For this review, take the finished solid that the model builds, in its own axes (mm). Face numbers are marked on the shaded views. A direction names the side the tool comes from. Coordinates: 2 decimals unless noted, no trailing zeros. Loops run counter-clockwise (first coordinate to the right, second up) from the corner with the lowest first, then second, coordinate; pieces in that order, holes last. Notation, with made-up numbers: (57.25, -14) -> (74.25, -14) arc R26 cw to (74.25, 4) -> close; hole circle Ø1 at (45, 57.5). An arc over 180 degrees is marked (long way). One line per item, written item: value.
from build123d import *

# Parameters (mm, degrees)
SKETCH1_W                   = 82.55
SKETCH1_H                   = 69.85
BOSS_EXTRUDE1_DEPTH         = 19.05
F_3_8_CLEARANCE_HOLE1_D     = 10.31875
F_3_8_CLEARANCE_HOLE1_DEPTH = 38.1
F_3_8_CLEARANCE_HOLE1_TIP   = 3.100065256
F_3_8_CLEARANCE_HOLE2_D     = 10.31875
F_3_8_CLEARANCE_HOLE2_DEPTH = 38.1
F_3_8_CLEARANCE_HOLE2_TIP   = 3.100065256
CUT_EXTRUDE2_START          = -19.05
SKETCH6_R                   = 7.3421875
CUT_EXTRUDE2_DEPTH          = 28.448
CUT_EXTRUDE4_START          = -19.05
SKETCH7_R                   = 12.7254
CUT_EXTRUDE4_DEPTH          = 2.8194
CUT_EXTRUDE6_START          = -19.05
SKETCH8_R                   = 7.3421875
CUT_EXTRUDE6_DEPTH          = 28.448
CUT_EXTRUDE8_START          = -19.05
SKETCH9_R                   = 12.7254
CUT_EXTRUDE8_DEPTH          = 2.8194
CUT_EXTRUDE10_START         = 41.275
SKETCH10_R                  = 7.3421875
CUT_EXTRUDE10_DEPTH         = 60.452


with BuildPart() as part:
    # Sketch1 → Boss-Extrude1 (new, symmetric)
    with BuildSketch(Plane(origin=(0, 0, 0), x_dir=(0, 1, 0), z_dir=(0, 0, 1))):
        Rectangle(SKETCH1_W, SKETCH1_H)
    extrude(amount=BOSS_EXTRUDE1_DEPTH, both=True)

    # 3/8 Clearance Hole1
    with Locations(Plane(origin=(0, 0, -19.05), x_dir=(-1, 0, 0), z_dir=(0, 0, -1))):
        with Locations((-23.876, -30.226)):
            Hole(F_3_8_CLEARANCE_HOLE1_D / 2, depth=F_3_8_CLEARANCE_HOLE1_DEPTH)
            with Locations((0, 0, -(F_3_8_CLEARANCE_HOLE1_DEPTH + F_3_8_CLEARANCE_HOLE1_TIP / 2))):  # 118° drill point
                Cone(0, F_3_8_CLEARANCE_HOLE1_D / 2, F_3_8_CLEARANCE_HOLE1_TIP, mode=Mode.SUBTRACT)

    # 3/8 Clearance Hole2
    with Locations(Plane(origin=(0, 0, -19.05), x_dir=(-1, 0, 0), z_dir=(0, 0, -1))):
        with Locations((-23.876, 30.099), (23.749, -30.226), (23.749, 30.099)):
            Hole(F_3_8_CLEARANCE_HOLE2_D / 2, depth=F_3_8_CLEARANCE_HOLE2_DEPTH)
            with Locations((0, 0, -(F_3_8_CLEARANCE_HOLE2_DEPTH + F_3_8_CLEARANCE_HOLE2_TIP / 2))):  # 118° drill point
                Cone(0, F_3_8_CLEARANCE_HOLE2_D / 2, F_3_8_CLEARANCE_HOLE2_TIP, mode=Mode.SUBTRACT)

    # Sketch6 → Cut-Extrude2 (cut)
    with BuildSketch(Plane(origin=(0, 0, 0), x_dir=(0, 1, 0), z_dir=(0, 0, 1)).offset(CUT_EXTRUDE2_START)):
        with Locations(Location((-17.653, -0.127, 0), (0, 0, 270))):
            Circle(SKETCH6_R)
    extrude(amount=CUT_EXTRUDE2_DEPTH, mode=Mode.SUBTRACT)

    # Sketch7 → Cut-Extrude4 (cut)
    with BuildSketch(Plane(origin=(0, 0, 0), x_dir=(0, 1, 0), z_dir=(0, 0, 1)).offset(CUT_EXTRUDE4_START)):
        with Locations(Location((-17.653, -0.127, 0), (0, 0, 270))):
            Circle(SKETCH7_R)
    extrude(amount=CUT_EXTRUDE4_DEPTH, mode=Mode.SUBTRACT)

    # Sketch8 → Cut-Extrude6 (cut)
    with BuildSketch(Plane(origin=(0, 0, 0), x_dir=(0, 1, 0), z_dir=(0, 0, 1)).offset(CUT_EXTRUDE6_START)):
        with Locations(Location((17.399, -0.127, 0), (0, 0, 270))):
            Circle(SKETCH8_R)
    extrude(amount=CUT_EXTRUDE6_DEPTH, mode=Mode.SUBTRACT)

    # Sketch9 → Cut-Extrude8 (cut)
    with BuildSketch(Plane(origin=(0, 0, 0), x_dir=(0, 1, 0), z_dir=(0, 0, 1)).offset(CUT_EXTRUDE8_START)):
        with Locations(Location((17.399, -0.127, 0), (0, 0, 270))):
            Circle(SKETCH9_R)
    extrude(amount=CUT_EXTRUDE8_DEPTH, mode=Mode.SUBTRACT)

    # Sketch10 → Cut-Extrude10 (cut)
    with BuildSketch(Plane(origin=(0, 0, 0), x_dir=(-1, 0, 0), z_dir=(0, 1, 0)).offset(CUT_EXTRUDE10_START)):
        with Locations((-0.127, 0)):
            Circle(SKETCH10_R)
    extrude(amount=-CUT_EXTRUDE10_DEPTH, mode=Mode.SUBTRACT)


solid = part.part
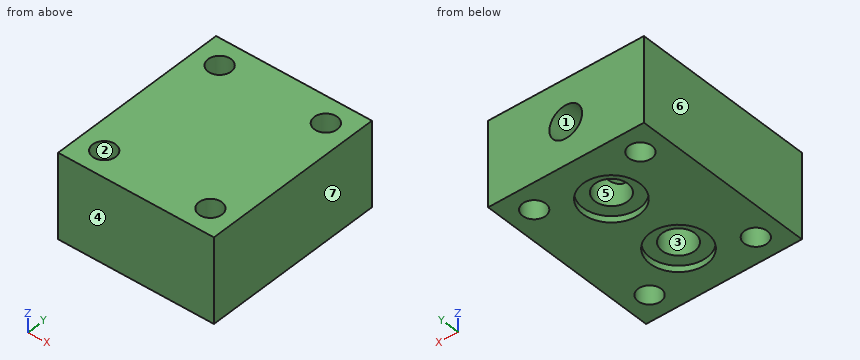
1. The part is to be moulded in two halves that separate along X. For the marked faces 4, 5, 6 and 7, say which applies: pulls with the +X half, pulls with the -X half, needs draft (parallel to the pull), parting line crosses it, or undercut.
Return value:
face 4: needs draft
face 5: undercut
face 6: pulls with the -X half
face 7: pulls with the +X half
2. For the marked faces 1, 2 and 3, list the 3-axis set-ups (+Z, -Z, +X, -X, +Y, -Y) from which the entire face can be reached by the end or side of a thin tool; tool diameter is ignored.
Return value:
face 1: +Y
face 2: +Z, -Z
face 3: -Z
3. Take a section at D-D, the plane z = -13.5. Give the boundary of the cut face in (x, y) (3 decimals).
Return value:
outline: (-34.925, -41.275) -> (34.925, -41.275) -> (34.925, 41.275) -> (-34.925, 41.275) -> close; hole circle Ø10.319 at (-23.749, -30.226); hole circle Ø10.319 at (-23.749, 30.099); hole circle Ø14.684 at (0.127, -17.653); hole circle Ø14.684 at (0.127, 17.399); hole circle Ø10.319 at (23.876, -30.226); hole circle Ø10.319 at (23.876, 30.099)
4. Take a section at A-A, the plane y = 33. Give the boundary of the cut face in (x, z) (3 decimals), and give its area (3 significant figures).
Return value:
outline: (-34.925, -19.05) -> (-28.016, -19.05) -> (-28.016, 19.05) -> (-34.925, 19.05) -> close; (-19.482, -19.05) -> (19.609, -19.05) -> (19.609, 19.05) -> (-19.482, 19.05) -> close; (28.143, -19.05) -> (34.925, -19.05) -> (34.925, 19.05) -> (28.143, 19.05) -> close; hole circle Ø14.684 at (0.127, 0)
area: 1,840 mm2
5. Take a section at B-B, the plane x = 6. Give the boundary of the cut face in (y, z) (3 decimals), and give its area (3 significant figures).
Return value:
outline: (-41.275, -19.05) -> (-28.942, -19.05) -> (-28.942, -16.231) -> (-22.059, -16.231) -> (-22.059, 9.398) -> (-13.247, 9.398) -> (-13.247, 4.406) -> (12.993, 4.406) -> (12.993, 9.398) -> (21.805, 9.398) -> (21.805, 4.406) -> (41.275, 4.406) -> (41.275, 19.05) -> (-41.275, 19.05) -> close; (-13.247, -16.231) -> (-6.364, -16.231) -> (-6.364, -19.05) -> (6.11, -19.05) -> (6.11, -16.231) -> (12.993, -16.231) -> (12.993, -4.406) -> (-13.247, -4.406) -> close; (21.805, -16.231) -> (28.688, -16.231) -> (28.688, -19.05) -> (41.275, -19.05) -> (41.275, -4.406) -> (21.805, -4.406) -> close
area: 2,160 mm2
6. Insertion check: pin 1 Ø9.5 at (x, y) = (-23.749, -30.226) entering from +Z; pin 2 Ø4.5 at (x, y) = (-0.5, -20) entering from -Z; pin 3 Ø15.5 at (x, y) = (0.127, 17.399) entering from -Z; pin 4 Ø9 at (x, z) = (0.127, 0) entering from +Y. Each pin has a flat end and moves straight along its axis. Give the tip position at first contact, or say it passes through.
Return value:
pin 1: passes through
pin 2: stops at z = 9.4
pin 3: stops at z = -16.23
pin 4: stops at y = -23.45
7. Take a section at C-C, the plane z = -3. Give the boundary of the cut face in (x, y) (3 decimals), and give its area (3 significant figures).
Return value:
outline: (-34.925, -41.275) -> (34.925, -41.275) -> (34.925, 41.275) -> (6.828, 41.275) -> (6.828, 20.399) arc R7.342 cw to (6.828, 14.399) -> (6.828, -14.653) arc R7.342 cw (long way) to (-6.574, -14.653) -> (-6.574, 14.399) arc R7.342 cw to (-6.574, 20.399) -> (-6.574, 41.275) -> (-34.925, 41.275) -> close; hole circle Ø10.319 at (-23.749, -30.226); hole circle Ø10.319 at (-23.749, 30.099); hole circle Ø10.319 at (23.876, -30.226); hole circle Ø10.319 at (23.876, 30.099)
area: 4,550 mm2
8. To check wall thickness, follow probe 1 along Y at (x, z) = (-19.5, 5) (3 decimals); probe 2 along Y at (x, z) = (-25.5, -13) (3 decimals); probe 3 along Z at (x, y) = (-6.5, -20). State the ranges of each line that lie inside material, in increasing order. Write a range as from..to.
Return value:
probe 1: y = -41.275..-33.153, -27.299..27.172, 33.026..41.275
probe 2: y = -41.275..-35.079, -25.373..25.246, 34.952..41.275
probe 3: z = 9.4..19.05
